from build123d import *

# Parameters (mm, degrees)
F0_W     = 2
F0_H     = 2
F1_DEPTH = 1.5
F2_R     = 0.5


with BuildPart() as f1:
    # F0 (on Right) → F1 (new body, symmetric)
    with BuildSketch(Plane.YZ):
        with BuildLine():
            Line((-50, 0), (0, 0))
            Line((0, 0), (0, 4))
            Line((0, 4), (-57, 4))
            ThreePointArc((-57, 4), (-59.12132, 3.12132), (-60, 1))
            Line((-60, 1), (-60, 0))
            Line((-60, 0), (-56, 0))
            Line((-56, 0), (-52, 0))
            Line((-52, 0), (-50, 0))
        make_face()
        with Locations((-51, -1)):
            Rectangle(F0_W, F0_H)
        with BuildLine():
            Line((-50, -2.5), (-50, -2))
            Line((-50, -2), (-52, -2))
            Line((-52, -2), (-52, -3))
            Line((-52, -3), (-50.5, -3))
            ThreePointArc((-50.5, -3), (-50.146447, -2.853553), (-50, -2.5))
        make_face()
        with BuildLine():
            Line((-56, -2.5), (-56, 0))
            Line((-56, 0), (-60, 0))
            Line((-60, 0), (-60, -1))
            ThreePointArc((-60, -1), (-59.414214, -2.414214), (-58, -3))
            Line((-58, -3), (-56.5, -3))
            ThreePointArc((-56.5, -3), (-56.146447, -2.853553), (-56, -2.5))
        make_face()
        with BuildLine():
            Line((-52, -3), (-52, -2))
            ThreePointArc((-52, -2), (-52.5, -2.5), (-52, -3))
        make_face()
    extrude(amount=F1_DEPTH, both=True)

    # F2
    f2_edges = [f1.edges().sort_by_distance(p)[0] for p in [
        (0, -56, 0),
        (0, -52, 0),
        (0, -50, 0),
    ]]
    fillet(f2_edges, radius=F2_R)

    # F3: F1 across face


with BuildPart() as f1_1:
    add(f1.part)
    add(f1.part.mirror(Plane(origin=(0, 0, 2), x_dir=(-1, 0, 0), z_dir=(0, 1, 0))))


solid = f1_1.part
Read the model definition and answer for the solid it produces. Units are mm, in the model's axes. A direction names the side the tool comes from. Round coordinates to 2 decimals unless told otherwise and drop trailing zeros. Order: outer loops, then holes, each group sorted by start corner. A loop starts at its lowest first (then second) coordinate and runs counter-clockwise, first axis right, second up. Notation, with made-up numbers: (88, 49.5) - (105, 49.5) arc R23 ccw to (105, 62.5) - close; hole circle Ø3 at (55.5, 84.5). An arc over 180 degrees is marked (long way). Use one line per item in the form item = value. Start each with the question number.
(1) For faces 5 (the face through (0, 54, 0)), 6 (the face through (0, -1, 4)), determine the directions among +Z, -Z, +X, -X, +Y, -Y from which every point of the face is accessible in a straight line to the end or side of a thin tool.
(2) Flat-ended cylindrical pins translate along their axes: pin 1 Ø1.5 at (x, y) = (-1, -20.5) entering from -Z; pin 2 Ø1.6 at (x, z) = (0.5, -2) entering from -Y; pin 3 Ø0.8 at (x, z) = (-0.5, -1.5) entering from +Y. Find the tip coordinate at first contact, or state that the pin passes through.
(3) Find the intervals of material crossed by line 1 along Y through (x, z) = (-0.9, -1); line 2 along Y through (x, z) = (-0.6, -0.25); line 3 along Z through (x, y) = (1.25, -39.5), in increasing order. Write a range as from..to.
(4) The part is cut by section B-B (y = -47.5). Give the vertices of the cut face in (x, z), then the cut area to 3 significant figures.
(5) Determine the mould class of faces 1 (the face through (0, -54, 0)), 2 (the face through (1.5, 1, 2)), 3 (the face through (0, 60, 0)), 4 (the face through (0.02, -59.1, 3.14)) for opening direction Y: +Y half, -Y half, draft (parallel to the pull), parting line (faces both ways), or undercut.
Checked values:
q1.face_5 = -Z, +X, -X
q1.face_6 = +Z, +X, -X, +Y, -Y
q2.pin_1 = 0
q2.pin_2 = -59.99
q2.pin_3 = 60
q3.line_1 = -60..-56, -52..-50, 50..52, 56..60
q3.line_2 = -60..-55.93, -52.07..-49.93, 49.93..52.07, 55.93..60
q3.line_3 = 0..4
q4.outline = (-1.5, 0) - (1.5, 0) - (1.5, 4) - (-1.5, 4) - close
q4.area = 12.0 mm^2
q5.face_1 = undercut
q5.face_2 = draft
q5.face_3 = +Y half
q5.face_4 = -Y half
